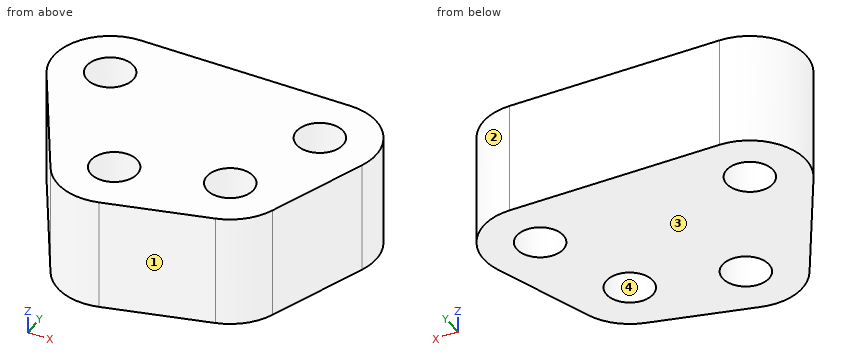
```python
from build123d import *

# Parameters (mm, degrees)
BOSS_EXTRU_1_DEPTH = 8
TROU_TARAUD_M41_D  = 3.3


with BuildPart() as part:
    # Esquisse1 → Boss.-Extru.1 (new body)
    with BuildSketch(Plane.XY):
        with BuildLine():
            Line((-15, 4), (0, 4))
            ThreePointArc((0, 4), (3.276608177, 2.294305745), (3.758770483, -1.368080573))
            Line((3.758770483, -1.368080573), (1.193619408, -8.415775229))
            ThreePointArc((1.193619408, -8.415775229), (0.137209756, -9.996804003), (-1.529874895, -10.911397961))
            Line((-1.529874895, -10.911397961), (-8.774922628, -12.85270265))
            ThreePointArc((-8.774922628, -12.85270265), (-11.340932538, -12.684517475), (-13.274300423, -10.988999345))
            Line((-13.274300423, -10.988999345), (-18.464101615, -2))
            ThreePointArc((-18.464101615, -2), (-18.464101615, 2), (-15, 4))
        make_face()
    extrude(amount=BOSS_EXTRU_1_DEPTH)

    # Trou taraudé M41 (through all)
    with Locations(Plane(origin=(0, 0, 0), x_dir=(1, 0, 0), z_dir=(0, 0, -1))):
        with Locations((-15, 0), (0, 0), (-2.565151075, 7.047694656), (-9.810198808, 8.988999345)):
            Hole(TROU_TARAUD_M41_D / 2)


solid = part.part
```
The model under review builds one solid part; all positions refer to its coordinate system, in mm. Face numbers are marked on the shaded views. Round coordinates to 2 decimals unless told otherwise and drop trailing zeros. Write each loop counter-clockwise with the first axis right and the second up, starting at its lowest first coordinate (ties: lowest second). Pieces come first, ordered by that corner, then holes. Notation, with made-up numbers: (10, -6.5) - (35, -6.5) arc R17 cw to (35, 13.5) - close; hole circle Ø9 at (57, -39). An arc over 180 degrees is marked (long way). One line per question, with ' | ' between items.
Item 1: Add section B-B, the plane x = -16. Give the boundary of the cut face in (y, z), then the cut area to 3 significant figures.
Resolved:
outline: (-6.27, 0) - (-1.31, 0) - (-1.31, 8) - (-6.27, 8) - close; (1.31, 0) - (3.87, 0) - (3.87, 8) - (1.31, 8) - close | area: 60.1 mm2
Item 2: Add section C-C, the plane z = 2.5. Give the boundary of the cut face in (x, y), then the cut area to 3 significant figures.
Resolved:
outline: (-18.46, -2) - (-13.27, -10.99) arc R4 ccw to (-8.77, -12.85) - (-1.53, -10.91) arc R4 ccw to (1.19, -8.42) - (3.76, -1.37) arc R4 ccw to (0, 4) - (-15, 4) arc R4 ccw to start; hole circle Ø3.3 at (-15, 0); hole circle Ø3.3 at (-9.81, -8.99); hole circle Ø3.3 at (-2.57, -7.05); hole circle Ø3.3 at (0, 0) | area: 268 mm2
Item 3: Add section D-D, the plane x = -7.75. Give the boundary of the cut face in (y, z), then the cut area to 3 significant figures.
Resolved:
outline: (-12.58, 0) - (4, 0) - (4, 8) - (-12.58, 8) - close | area: 133 mm2
Item 4: For P1, Ø1, axis at y = -9, z = 3.5, coming from the +X side; P2, Ø4, axis at y = 2.5, z = 1, coming from the -X side, all flat-tipped, find the tip position at first contact; note any pin that passes through.
Resolved:
P1: stops at x = 1.16 | P2: stops at x = -18.97
Item 5: The part is to be moulded in two halves that separate along Y. For the marked faces 1, 2, 3 and 4, say which applies: pulls with the +Y half, pulls with the -Y half, needs draft (parallel to the pull), parting line crosses it, or undercut.
Resolved:
face 1: pulls with the -Y half | face 2: parting line crosses it | face 3: needs draft | face 4: undercut
Item 6: Add section A-A, the plane y = 0. Give the boundary of the cut face in (x, z).
Resolved:
outline: (-19, 0) - (-16.65, 0) - (-16.65, 8) - (-19, 8) - close; (-13.35, 0) - (-1.65, 0) - (-1.65, 8) - (-13.35, 8) - close; (1.65, 0) - (4, 0) - (4, 8) - (1.65, 8) - close
Item 7: To check wall thickness, follow probe 1 along X at (y, z) = (0.25, 1); probe 2 along X at (y, z) = (-6, 6); probe 3 along X at (y, z) = (-10.25, 4.25). State the ranges of each line that lie inside material, in increasing order.
Resolved:
probe 1: x = -18.99 to -16.63, -13.37 to -1.63, 1.63 to 3.99 | probe 2: x = -16.15 to -3.84, -1.29 to 2.07 | probe 3: x = -13.7 to -10.87, -8.75 to -0.17
